Build history of the part. All positions in model axes, mm. A direction names the side the tool comes from. Round coordinates to 2 decimals unless told otherwise and drop trailing zeros. Loops run counter-clockwise (first coordinate to the right, second up) from the corner with the lowest first, then second, coordinate; pieces in that order, holes last. Notation, with made-up numbers: (46.25, 11) - (73.25, 11) arc R18 cw to (73.25, 18) - close; hole circle Ø4 at (43, -29.75). An arc over 180 degrees is marked (long way). Use one line per item in the form item = value. Start each with the question number.
Q1. Saw through at C-C (z = 2). Count the separate pieces of the cut face and the enclosed holes in it, then the cut area to 3 significant figures.
Q2. 3-axis set-ups, long thin cutter, end or side, ignore diameter. For faces 1 (the face through (99.344, 106.114, 3.131)), 2 (the face through (155, 146.906, 3)): which of +Z, -Z, +X, -X, +Y, -Y reach the whole face in a straight line?
Q3. Pin check, flat tip, straight feed: pin 1 (3 mm diameter, centred on x = 229.84, y = 61.42, fed in from +Z). Stop position of the tip, or through.
Q4. Saw through at B-B (x = 159). Give the cut face in (y, z).
Q5. Drill centre lines: line 1 (X direction, y = 67.5, z = 4.75); line 2 (X direction, y = 108, z = 3.5); line 3 (X direction, y = 62, z = 2.75). Where is each one in solid material? Low to high.
Q6. Saw through at D-D (x = 132). Give the cut face in (y, z), then the cut area to 3 significant figures.
Q7. Mould opens along X. For faces 3 (the face through (166.03, 21.11, 3.13)), 4 (the face through (257.611, 69, 3)), 5 (the face through (157, -11.844, 3)) say: released by +X, released by -X, zero draft, split by the parting line, or undercut.
Q8. Saw through at A-A (y = 25.4). Give the cut face in (x, z).
Autodesk Inventor part; units mm, degrees
ref_plane "YZ Plane" through (0, 0, 0) normal (1, 0, 0) x (0, 1, 0)
ref_plane "XZ Plane" through (0, 0, 0) normal (0, 1, 0) x (-1, 0, 0)
ref_plane "XY Plane" through (0, 0, 0) normal (0, 0, 1) x (1, 0, 0)
sketch "Sketch1" plane through (0, 0, 0) normal (0, 0, 1) x (1, 0, 0)
  line L0 (0, 0) -> (304.8, 0) construction
  line L1 (304.8, 0) -> (304.8, 50.8) construction
  line L2 (304.8, 50.8) -> (0, 50.8) construction
  line L3 (0, 50.8) -> (0, 0) construction
  circle A0 centre (152.4, 25.4) radius 14.2875
  circle A1 centre (152.4, 25.4) radius 30.48 construction
  circle A2 centre (152.4, 25.4) radius 22.225 construction
  line L4 (152.4, 25.4) -> (138.5082, 62.9697) construction
  circle A3 centre (138.5082, 62.9697) radius 9.525 construction
  circle A4 centre (138.5082, 62.9697) radius 17.78 construction
  circle A5 centre (89.9711, 85.09) radius 31.75
  circle A6 centre (160.9785, 111.3458) radius 31.75
  circle A7 centre (220.6325, 85.09) radius 31.75
  line L5 (0, 50.8) -> (0, 53.34) construction
  line L6 (0, 53.34) -> (304.8, 53.34) construction
  line L7 (304.8, 53.34) -> (304.8, 50.8) construction
  circle A8 centre (138.5082, 62.9697) radius 21.59 construction
  circle A9 centre (152.4, 25.4) radius 46.99 construction
  circle A10 centre (152.4, 25.4) radius 50.8 construction
  arc A11 (84.9408, 79.3264) -> (90.9184, 92.6811) centre (89.9711, 85.09) ccw construction
  circle A12 centre (160.9785, 111.3458) radius 7.65 construction
  circle A13 centre (220.6325, 85.09) radius 7.65 construction
  circle A14 centre (160.9785, 111.3458) radius 9.1 construction
  line L8 (164.8287, 119.5911) -> (223.8692, 92.0215) construction
  line L9 (157.4988, 102.9373) -> (217.7073, 78.0214) construction
  circle A15 centre (138.5082, 62.9697) radius 22.9 construction
  line L10 (84.9408, 79.3264) -> (123.4503, 45.7166) construction
  line L11 (168.5483, 110.2412) -> (161.1682, 59.6633) construction
  line L12 (90.9184, 92.6811) -> (89.9711, 85.09) construction
  line L13 (89.9711, 85.09) -> (84.9408, 79.3264) construction
  circle A16 centre (126.192, 96.2783) radius 3.175
  circle A17 centre (126.192, 96.2783) radius 7.9375 construction
  line L14 (90.9184, 92.6811) -> (125.2091, 88.4019) construction
  line L15 (132.0626, 90.936) -> (155.3205, 116.4945) construction
  line L16 (155.3205, 116.4945) -> (160.9785, 111.3458) construction
  line L17 (168.5483, 110.2412) -> (160.9785, 111.3458) construction
  line L18 (138.5082, 62.9697) -> (126.192, 96.2783) construction
  line L19 (89.9711, 85.09) -> (160.9785, 111.3458) construction
  line L20 (152.4, 25.4) -> (89.9711, 85.09) construction
  line L21 (152.4, 25.4) -> (160.9785, 111.3458) construction
  circle A18 centre (126.192, 96.2783) radius 9.2075 construction
  circle A19 centre (126.192, 96.2783) radius 6.1595 construction
  arc A20 (90.9184, 92.6811) -> (84.9408, 79.3264) centre (89.9711, 85.09) ccw construction
  line L22 (160.9785, 111.3458) -> (220.6325, 85.09) construction
  circle A21 centre (160.9785, 111.3458) radius 25.4 construction
  circle A22 centre (220.6325, 85.09) radius 25.4 construction
  line L23 (102.9424, 114.0695) -> (76.9998, 56.1105) construction
  circle A23 centre (89.9711, 85.09) radius 25.4 construction
  line L24 (209.1281, 114.6824) -> (232.1368, 55.4976) construction
  circle A24 centre (160.9785, 111.3458) radius 10.16
  line L25 (54.4111, 146.9058) -> (257.6111, 146.9058)
  line L26 (257.6111, 146.9058) -> (257.6111, -11.8442)
  line L27 (257.6111, -11.8442) -> (54.4111, -11.8442)
  line L28 (54.4111, -11.8442) -> (54.4111, 146.9058)
  circle A25 centre (138.5082, 62.9697) radius 11.1125
  arc A26 (225.0295, 75.8783) -> (218.6208, 95.1612) centre (221.8252, 85.5197) ccw
  line L29 (219.4627, 84.6013) -> (229.8359, 61.416) construction
  line L30 (221.8252, 85.5197) -> (229.8359, 61.416) construction
  line L31 (219.4627, 84.6013) -> (209.0895, 107.7866) construction
  line L32 (221.8252, 85.5197) -> (213.8144, 109.6234) construction
  arc A27 (208.117, 109.9602) -> (210.062, 105.6129) centre (209.0895, 107.7866) ccw
  arc A28 (214.5654, 107.3637) -> (213.0634, 111.8831) centre (213.8144, 109.6234) ccw
  arc A29 (214.5654, 107.3637) -> (210.062, 105.6129) centre (229.8359, 61.416) ccw
  arc A30 (213.0634, 111.8831) -> (208.117, 109.9602) centre (229.8359, 61.416) ccw
  line L33 (209.0895, 107.7866) -> (208.117, 109.9602) construction
  line L34 (213.8144, 109.6234) -> (213.0634, 111.8831) construction
  arc A31 (218.6208, 95.1612) -> (215.3134, 93.8754) centre (229.8359, 61.416) ccw
  arc A32 (225.0295, 75.8783) -> (223.612, 75.3272) centre (229.8359, 61.416) ccw
  line L35 (102.6358, 107.1803) -> (91.1149, 84.5434) construction
  line L36 (79.5941, 61.9064) -> (88.8014, 85.5789) construction
  arc A33 (98.8719, 111.4706) -> (97.1455, 107.0321) centre (98.0087, 109.2513) ccw
  arc A34 (101.5557, 105.0581) -> (103.7158, 109.3025) centre (102.6358, 107.1803) ccw
  arc A35 (101.5557, 105.0581) -> (97.1455, 107.0321) centre (79.5941, 61.9064) ccw
  line L37 (98.0087, 109.2513) -> (98.8719, 111.4706) construction
  line L38 (102.6358, 107.1803) -> (103.7158, 109.3025) construction
  arc A36 (103.7158, 109.3025) -> (98.8719, 111.4706) centre (79.5941, 61.9064) ccw
  arc A37 (215.3134, 93.8754) -> (223.612, 75.3272) centre (219.4627, 84.6013) ccw
  arc A38 (86.5066, 75.4886) -> (95.7233, 93.5981) centre (91.1149, 84.5434) ccw
  line L39 (88.8014, 85.5789) -> (98.0087, 109.2513) construction
  line L40 (91.1149, 84.5434) -> (79.5941, 61.9064) construction
  arc A39 (86.5066, 75.4886) -> (85.1185, 76.1099) centre (79.5941, 61.9064) ccw
  arc A40 (95.7233, 93.5981) -> (92.4843, 95.0479) centre (79.5941, 61.9064) ccw
  arc A41 (92.4843, 95.0479) -> (85.1185, 76.1099) centre (88.8014, 85.5789) ccw
  line L41 (160.9785, 111.3458) -> (137.7306, 121.5779) construction
  point P0 (184.2263, 101.1136)
  point P1 (211.429, 108.764)
  point P2 (100.3481, 108.2736)
  dimension "d1" = 50.8
  dimension "d2" = 28.575
  dimension "d3" = 25.4
  dimension "d4" = 152.4
  dimension "d7" = 60.96
  dimension "d8" = 44.45
  dimension "d9" = 19.05
  dimension "d10" = 35.56
  dimension "d11" = 40.0558
  dimension "d12" = 63.5
  dimension "d13" = 63.5
  dimension "d14" = 63.5
  dimension "d15" = 2.54
  dimension "d16" = 304.8
  dimension "d17" = 43.18
  dimension "d18" = 93.98
  dimension "d19" = 101.6
  dimension "d21" = 15.3
  dimension "d22" = 15.3
  dimension "d23" = 15.3
  dimension "d24" = 18.2
  dimension "d29" = 45.8
  dimension "d30" = 146
  dimension "d31" = 6.35
  dimension "d32" = 15.875
  dimension "d33" = 146
  dimension "d35" = 18.415
  dimension "d37" = 12.319
  dimension "d38" = 65.1764
  dimension "d40" = 50.8
  dimension "d41" = 50.8
  dimension "d42" = 17
  dimension "d43" = 17
  dimension "d44" = 50.8
  dimension "d45" = 45
  dimension "d50" = 20.32
  dimension "d53" = 203.2
  dimension "d54" = 158.75
  dimension "d55" = 35.56
  dimension "d56" = 35.56
  dimension "d57" = 22.225
  dimension "d67" = 25.4
  dimension "d68" = 25.4
  dimension "d69" = 2.86
  dimension "d70" = 25.4
  dimension "d71" = 25.4
  dimension "d72" = 4.7625
  dimension "d75" = 2.86
  dimension "d80" = 4.7625
  dimension "d82" = 4.7625
  dimension "d83" = 50.8
  dimension "d84" = 50.8
  dimension "d85" = 10.16
  dimension "d97" = 48.4188
  dimension "d99" = 20.32
  dimension "d101" = 25.4
  dimension "d102" = 25.4
  dimension "d103" = 10.16
  dimension "d104" = 180
extrude "Extrusion2" add sketch "Sketch1" along normal blind 6.35 contours A5 | A6 | A7 | L25 L26 L27 L28
hole "Hole2" at (79.5941, 61.9064, 0) at (229.8359, 61.416, 0) at (184.2263, 101.1136, 0) at (137.7306, 121.5779, 0) direction (0, 0, 1) diameter 4.7625 end through all
equation "\"d2\" = BearingLargeOD"
equation "\"d7\" = Gear48tPD"
equation "\"d8\" = Gear35tPD"
equation "\"d9\" = Gear15tPD"
equation "\"d10\" = Gear28tPD"
equation "\"d11\" = 0.5 * Gear48tPD + 0.5 * Gear15tPD + MeshingClearance"
equation "\"d12\" = CimOD"
equation "\"d13\" = CimOD"
equation "\"d14\" = CimOD"
equation "\"d17\" = Gear28tPD + ClearanceDiameter"
equation "\"d18\" = WheelOD"
equation "\"d19\" = WheelClearance"
equation "\"Pulley48tPD\" = 45.8"
equation "\"Pulley19tPD\" = 18.2"
equation "\"Pulley16tPD\" = 15.3"
equation "\"Gear15tPD\" = 19.05"
equation "\"Gear35tPD\" = 44.45"
equation "\"Gear48tPD\" = 60.96"
equation "\"Gear28tPD\" = 35.56"
equation "\"BearingLargeOD\" = 28.575"
equation "\"BearingSmallOD\" = 22.225"
equation "\"MeshingClearance\" = 0.0508"
equation "\"CimOD\" = 63.5"
equation "\"WheelOD\" = 93.98"
equation "\"ClearanceDiameter\" = 7.62"
equation "\"WheelClearance\" = 101.6"
equation "\"TensioningBearingID\" = 6.35"
equation "\"TensioningBearingOD\" = 15.875"
equation "\"SpingClipClearance\" = 8.89"
equation "\"Pi\" = 79.79645"
properties part number "OutlineSketch1"
Report:
q1.separate_pieces = 1
q1.enclosed_holes = 12
q1.area = 30,000 mm²
q2.face_1 = +Z, -Z
q2.face_2 = +Z, -Z, +X, -X, +Y
q3.pin_1 = through
q4.outline = (-11.84, 0) - (12.73, 0) - (12.73, 6.35) - (-11.84, 6.35) - close; (38.07, 0) - (101.38, 0) - (101.38, 6.35) - (38.07, 6.35) - close; (121.31, 0) - (146.91, 0) - (146.91, 6.35) - (121.31, 6.35) - close
q5.line_1 = 54.41 to 128.36, 148.66 to 257.61
q5.line_2 = 54.41 to 95.98, 104.87 to 151.39, 170.57 to 206.72, 215.56 to 257.61
q5.line_3 = 54.41 to 77.21, 81.97 to 127.44, 149.58 to 227.53, 232.14 to 257.61
q6.outline = (-11.84, 0) - (53.96, 0) - (53.96, 6.35) - (-11.84, 6.35) - close; (71.98, 0) - (146.91, 0) - (146.91, 6.35) - (71.98, 6.35) - close
q6.area = 894 mm²
q7.face_3 = undercut
q7.face_4 = released by +X
q7.face_5 = zero draft
q8.outline = (54.41, 0) - (138.11, 0) - (138.11, 6.35) - (54.41, 6.35) - close; (166.69, 0) - (257.61, 0) - (257.61, 6.35) - (166.69, 6.35) - close
